Part print with two shaded views. Sizes in mm from the minimum x, y, z corner. Round coordinates to 2 decimals unless told otherwise and drop trailing zeros. Loops run counter-clockwise (first coordinate to the right, second up) from the corner with the lowest first, then second, coordinate; pieces in that order, holes last.
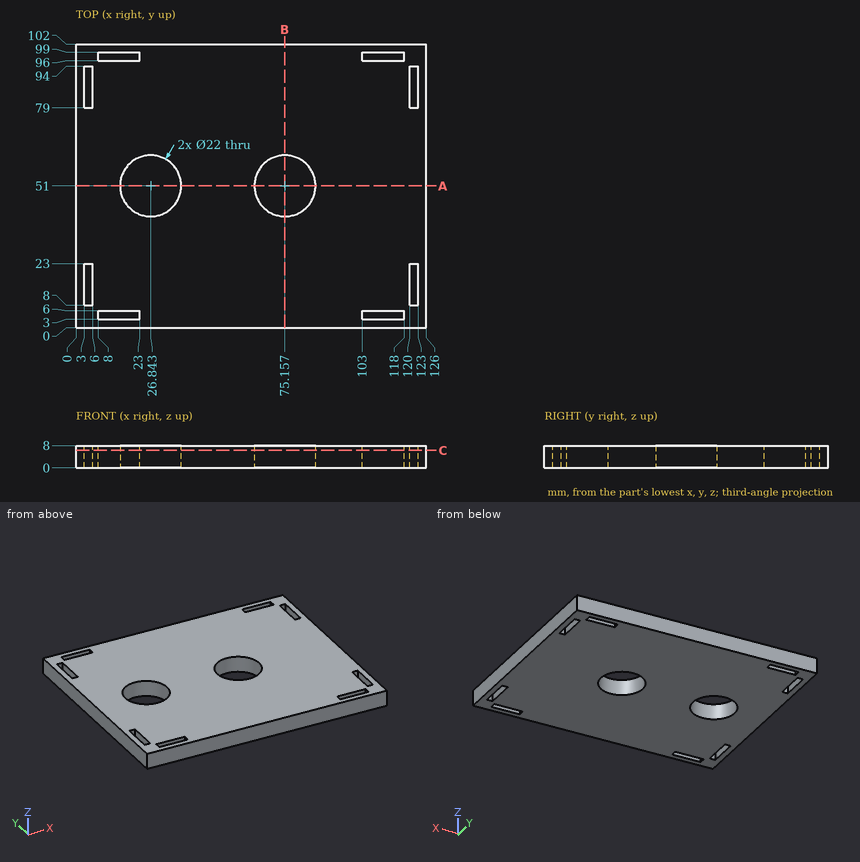
Item 1: Cut at B-B (x = 75). List the corners of the cut face in (y, z).
Verdict:
outline: (0, 0) - (40, 0) - (40, 8) - (0, 8) - close; (62, 0) - (102, 0) - (102, 8) - (62, 8) - close
Item 2: Cut at C-C (z = 6.25). State how many separate pieces and enclosed holes the cut face has, plus the area to 3 significant figures.
Verdict:
separate pieces: 1
enclosed holes: 10
area: 11,700 mm2
Item 3: Cut at A-A (y = 51). List the corners of the cut face in (x, z).
Verdict:
outline: (0, 0) - (15.84, 0) - (15.84, 8) - (0, 8) - close; (37.84, 0) - (64.16, 0) - (64.16, 8) - (37.84, 8) - close; (86.16, 0) - (126, 0) - (126, 8) - (86.16, 8) - close
Item 4: Wall check: L1, parallel to Y at x = 113.5, z = 1.5; L2, parallel to X at y = 82, z = 3.5; L3, parallel to X at y = 52, z = 4.25. Give the ranges that are in metal, low to high.
Verdict:
L1: y = 0 to 3, 6 to 96, 99 to 102
L2: x = 0 to 3, 6 to 120, 123 to 126
L3: x = 0 to 15.89, 37.8 to 64.2, 86.11 to 126
